The listing builds one solid part. Answer for the finished solid, in the listing's coordinates (mm). A direction names the side the tool comes from. Coordinates: 2 decimals unless noted, no trailing zeros. Write each loop counter-clockwise with the first axis right and the second up, starting at its lowest first coordinate (ties: lowest second). Pieces come first, ordered by that corner, then holes. Notation, with made-up numbers: M 1.5,0.5 L 48.5,0.5 A21 ccw 48.5,6.5 Z; hole C -18.5,-21 d9. An arc over 180 degrees is marked long. Write item = value, one per line. Start each with the question number.
```python
from build123d import *

# Parameters (mm, degrees)
F0_R     = 21.5
F1_DEPTH = 58
F2_R     = 15
F3_DEPTH = 46
F4_SIZE2 = 15
F4_SIZE  = 40


with BuildPart() as f1:
    # F0 (on Top) → F1 (new body)
    with BuildSketch(Plane.XY):
        Circle(F0_R)
    extrude(amount=F1_DEPTH)

    # F2 (on face) → F3 (join)
    with BuildSketch(Plane.XY.offset(58)):
        Circle(F2_R)
    extrude(amount=F3_DEPTH)

    # F4
    f4_edges = [f1.edges().sort_by_distance(p)[0] for p in [
        (-21.5, 0, 0),
    ]]
    chamfer(f4_edges, length=F4_SIZE, length2=F4_SIZE2)


solid = f1.part
```
1. The part is cut by section A-A, the plane y = 0. Write down the section's boundary in (x, z), and give its area (3 significant figures).
2. For faces 1 (the face through (-14.985, 0.66, 80.678)), 2 (the face through (-2.799, 21.317, 48.874)), determine the directions among +Z, -Z, +X, -X, +Y, -Y from which every point of the face is accessible in a straight line to the end or side of a thin tool.
3. The part is cut by section C-C, the plane z = 82. Write down the section's boundary in (x, y).
4. Straight lines are drawn through the part: L1, parallel to Y at x = 11, z = 47; L2, parallel to X at y = -17.5, z = 53; L3, parallel to X at y = -14, z = 54.5. For each, find the intervals that lie inside material, in ascending order. Write a range as [from, to].
5. This flat-tipped pin is pushed along its axis until it touches: pin 1 (6 mm diameter, centred on y = 9, z = 15, fed in from +X). Where does it stop, or does it pass through?
Solution:
q1.outline = M -21.5,40 L -6.5,0 L 6.5,0 L 21.5,40 L 21.5,58 L 15,58 L 15,104 L -15,104 L -15,58 L -21.5,58 Z
q1.area = 3,270 mm^2
q2.face_1 = +Z
q2.face_2 = +Z, -Z
q3.outline = C 0,0 d30
q4.L1 = [-18.47, 18.47]
q4.L2 = [-12.49, 12.49]
q4.L3 = [-16.32, 16.32]
q5.pin_1 = 10.97
